```python
from build123d import *

# Parameters (mm, degrees)
SKETCH1_W           = 40
SKETCH1_H           = 7
BOSS_EXTRUDE1_DEPTH = 40
CUT_EXTRUDE1_DEPTH  = 8
FILLET1_R           = 10
SKETCH5_W           = 5
SKETCH5_H           = 7
BOSS_EXTRUDE2_DEPTH = 20
FILLET2_R           = 7
FILLET3_R           = 3
SKETCH6_R           = 2
CUT_EXTRUDE2_DEPTH  = 41
SKETCH7_R           = 2
CUT_EXTRUDE3_DEPTH  = 23.5


with BuildPart() as part:
    # Sketch1 → Boss-Extrude1 (new body)
    with BuildSketch(Plane(origin=(0, 0, 0), x_dir=(0, 0, -1), z_dir=(1, 0, 0))):
        Rectangle(SKETCH1_W, SKETCH1_H)
    extrude(amount=BOSS_EXTRUDE1_DEPTH)

    # Sketch2 → Cut-Extrude1 (cut, through all)
    with BuildSketch(Plane(origin=(0, 3.5, 0), x_dir=(1, 0, 0), z_dir=(0, 1, 0))):
        with BuildLine():
            Line((5, 20), (35, 20))
            Line((35, 20), (35, 0))
            ThreePointArc((35, 0), (32.071067812, -7.071067812), (25, -10))
            Line((25, -10), (15, -10))
            ThreePointArc((15, -10), (7.928932188, -7.071067812), (5, 0))
            Line((5, 0), (5, 20))
        make_face()
    extrude(amount=-CUT_EXTRUDE1_DEPTH, mode=Mode.SUBTRACT)

    # Fillet1
    fillet1_edges = [part.edges().sort_by_distance(p)[0] for p in [
        (40, 0, 20),
        (0, 0, 20),
    ]]
    fillet(fillet1_edges, radius=FILLET1_R)

    # Sketch5 → Boss-Extrude2 (add)
    with BuildSketch(Plane.XY.offset(20)):
        with Locations((20, 0)):
            Rectangle(SKETCH5_W, SKETCH5_H)
    extrude(amount=BOSS_EXTRUDE2_DEPTH)

    # Fillet2
    fillet2_edges = [part.edges().sort_by_distance(p)[0] for p in [
        (17.5, 0, 20),
        (22.5, 0, 20),
    ]]
    fillet(fillet2_edges, radius=FILLET2_R)

    # Fillet3
    fillet3_edges = [part.edges().sort_by_distance(p)[0] for p in [
        (2.5, -3.5, -20),
        (2.5, 3.5, -20),
        (20, -3.5, 40),
        (20, 3.5, 40),
        (37.5, -3.5, -20),
        (37.5, 3.5, -20),
    ]]
    fillet(fillet3_edges, radius=FILLET3_R)

    # Sketch6 → Cut-Extrude2 (cut, through all)
    with BuildSketch(Plane(origin=(40, 0, 0), x_dir=(0, 0, -1), z_dir=(1, 0, 0))):
        with Locations((15, 0)):
            Circle(SKETCH6_R)
    extrude(amount=-CUT_EXTRUDE2_DEPTH, mode=Mode.SUBTRACT)

    # Sketch7 → Cut-Extrude3 (cut, through all)
    with BuildSketch(Plane(origin=(22.5, 0, 0), x_dir=(0, 0, -1), z_dir=(1, 0, 0))):
        with Locations((-36, 0)):
            Circle(SKETCH7_R)
    extrude(amount=-CUT_EXTRUDE3_DEPTH, mode=Mode.SUBTRACT)


solid = part.part
```
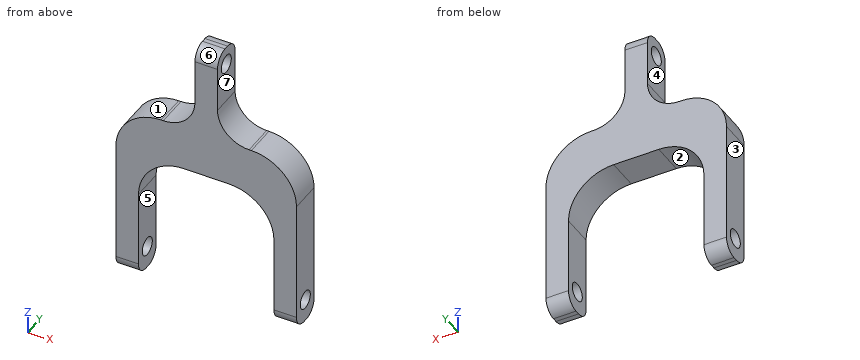
The listing builds one solid part. Answer for the finished solid, in the listing's coordinates (mm). Face numbers are marked on the shaded views. A direction names the side the tool comes from. Coordinates: 2 decimals unless noted, no trailing zeros. Loops run counter-clockwise (first coordinate to the right, second up) from the corner with the lowest first, then second, coordinate; pieces in that order, holes last. Notation, with made-up numbers: (81.25, 12.5) - (99.25, 12.5) arc R24 cw to (99.25, 35.5) - close; hole circle Ø1 at (27, 63). An arc over 180 degrees is marked (long way). Use a Markdown table: item, result. Add a question column.
1) Find the intervals of material crossed by line 1 (X direction, y = -3, z = -0.5); line 2 (Y direction, x = 37.3, z = -15); line 3 (X direction, y = 3.25, z = 3), in increasing order.
2) The mould has two halves that part along Z. Classify the marked faces 1, 2 and 3: released by +Z, released by -Z, zero draft, split by the parting line, or undercut.
3) The part is cut by section B-B, the plane z = -2. Give the vertices of the cut face in (x, y).
4) Given pin 1 (3 mm diameter, centred on x = 30.5, y = -1.5, fed in from -Z); pin 2 (1.5 mm diameter, centred on y = 1, z = 32.5, fed in from +X); pin 3 (0.6 mm diameter, centred on x = 30, y = -0.5, fed in from +Z); pin 4 (6 mm diameter, centred on x = 14, z = 31, fed in from +Y), each flat-ended and moving along its own axis, determine where each tip first touches the part or whether it passes through.
5) The part is cut by section D-D, the plane x = 32.5. Give the vertices of the cut face in (y, z).
6) For the marked faces 4, 5, 6 and 7, determine the directions among +Z, -Z, +X, -X, +Y, -Y from which every point of the face is accessible in a straight line to the end or side of a thin tool.
7) The part is cut by section A-A, the plane z = -15. Give the vertices of the cut face in (x, y).
8) The part is cut by section C-C, the plane z = 36. Give the vertices of the cut face in (x, y), and give its area (3 significant figures).
Here are the results:
| question | item | result |
|---|---|---|
| 1 | line 1 | x = 0 to 5, 35 to 40 |
| 1 | line 2 | y = -3.5 to -2, 2 to 3.5 |
| 1 | line 3 | x = 0 to 5.46, 34.54 to 40 |
| 2 | face 1 | released by +Z |
| 2 | face 2 | released by -Z |
| 2 | face 3 | zero draft |
| 3 | outline | (0, -3.5) - (5, -3.5) - (5, 3.5) - (0, 3.5) - close; (35, -3.5) - (40, -3.5) - (40, 3.5) - (35, 3.5) - close |
| 4 | pin 1 | stops at z = 7.14 |
| 4 | pin 2 | stops at x = 22.5 |
| 4 | pin 3 | stops at z = 20 |
| 4 | pin 4 | passes through |
| 5 | outline | (-3.5, 6.61) - (3.5, 6.61) - (3.5, 19.68) - (-3.5, 19.68) - close |
| 6 | face 4 | +Z, -X, +Y, -Y |
| 6 | face 5 | -Z, +Y, -Y |
| 6 | face 6 | +Z, +X, -X, -Y |
| 6 | face 7 | +Z, +X, +Y, -Y |
| 7 | outline | (0, -3.5) - (5, -3.5) - (5, -2) - (0, -2) - close; (0, 2) - (5, 2) - (5, 3.5) - (0, 3.5) - close; (35, -3.5) - (40, -3.5) - (40, -2) - (35, -2) - close; (35, 2) - (40, 2) - (40, 3.5) - (35, 3.5) - close |
| 8 | outline | (17.5, -3.5) - (22.5, -3.5) - (22.5, -2) - (17.5, -2) - close; (17.5, 2) - (22.5, 2) - (22.5, 3.5) - (17.5, 3.5) - close |
| 8 | area | 15.0 mm^2 |
